```python
from build123d import *

# Parameters (mm, degrees)
SKETCH_1_R      = 80.348196739
SKETCH_1_W      = 276.308595414
SKETCH_1_H      = 76.854046406
EXTRUDE_1_DEPTH = 100


with BuildPart() as part:
    # 草图1 → 凸台-拉伸1 (new body)
    with BuildSketch(Plane.XY):
        Circle(SKETCH_1_R)
        Rectangle(SKETCH_1_W, SKETCH_1_H)
    extrude(amount=EXTRUDE_1_DEPTH)


solid = part.part
```
Geometry: final body of the model. Coordinates: model frame, mm. A direction names the side the tool comes from. Round coordinates to 2 decimals unless told otherwise and drop trailing zeros. Write each loop counter-clockwise with the first axis right and the second up, starting at its lowest first coordinate (ties: lowest second). Pieces come first, ordered by that corner, then holes. Notation, with made-up numbers: (26.25, -8) -> (73.25, -8) arc R18 cw to (73.25, 13) -> close; hole circle Ø11 at (15.5, -17.75). An arc over 180 degrees is marked (long way). Use CSV: the item, a comma, the result in double quotes. Start each with the question number.
Q1. Section A-A (z = 80.5). Return loops of the section in (x, y), plus the area to 3 significant figures.
Q2. Line query: L1, parallel to Y at x = 96.5, z = 15.5; L2, parallel to X at y = -59.5, z = 41.5; L3, parallel to X at y = -45, z = 27.5. Output: solid intervals per line, ascending.
Q3. Section B-B (y = 53). Return loops of the section in (x, z).
Q4. Reachability of faces 1 (the face through (104, -38.427, 49)), 2 (the face through (-105, 38.427, 49)), 3 (the face through (104, 38.427, 49)), 4 (the face through (-2, 1, 100)) from +Z, -Z, +X, -X, +Y, -Y: full face, straight path, thin tool, end or side. Return the list, or none.
Q5. Pull-direction query (X, two-part tool) for faces 5 (the face through (-138.154, -1, 49)), 6 (the face through (-1.21, -80.34, 49.3)), 7 (the face through (138.154, -1, 49)), 8 (the face through (-105, -38.427, 49)); classes: pulls with the +X half, pulls with the -X half, needs draft (parallel to the pull), parting line crosses it, or undercut.
Q6. Section C-C (x = -32). Return loops of the section in (y, z).
Q7. First-contact query: pin 1 Ø20.5 at (x, z) = (-101.5, 27.5) entering from -Y; pin 2 Ø1.5 at (x, z) = (27.5, 64.5) entering from +Y; pin 3 Ø5 at (x, z) = (-7, 59.5) entering from -Y. Flat tips, straight axial feed; report the tip coordinate or a pass-through.
Result sheet:
1,outline,"(-138.15, -38.43) -> (-70.56, -38.43) arc R80.35 ccw to (70.56, -38.43) -> (138.15, -38.43) -> (138.15, 38.43) -> (70.56, 38.43) arc R80.35 ccw to (-70.56, 38.43) -> (-138.15, 38.43) -> close"
1,area,"29,700 mm²"
2,L1,"-38.43 to 38.43"
2,L2,"-54 to 54"
2,L3,"-66.56 to 66.56"
3,outline,"(-60.39, 0) -> (60.39, 0) -> (60.39, 100) -> (-60.39, 100) -> close"
4,face 1,"+Z, -Z, +X, -Y"
4,face 2,"+Z, -Z, -X, +Y"
4,face 3,"+Z, -Z, +X, +Y"
4,face 4,"+Z, +X, -X, +Y, -Y"
5,face 5,"pulls with the -X half"
5,face 6,"parting line crosses it"
5,face 7,"pulls with the +X half"
5,face 8,"needs draft"
6,outline,"(-73.7, 0) -> (73.7, 0) -> (73.7, 100) -> (-73.7, 100) -> close"
7,pin 1,"y = -38.43"
7,pin 2,"y = 75.76"
7,pin 3,"y = -80.22"
